from build123d import *

# Parameters (mm, degrees)
SKETCH_1_R          = 2.5
EXTRUDE_1_DEPTH     = 16
SKETCH_2_R          = 4.25
EXTRUDE_2_DEPTH     = 5
SKETCH_3_R          = 2
CUT_EXTRUDE_1_DEPTH = 3.4
CHAMFER_1_SIZE      = 0.8
FILLET_1_R          = 0.4
FILLET_2_R          = 0.2
CHAMFER_2_SIZE      = 0.4
CHAMFER_2_SIZE2     = 0.230940108
CUT_EXTRUDE_2_DEPTH = 2.8


with BuildPart() as part:
    # Эскиз1 → Вытянуть1 (new body)
    with BuildSketch(Plane(origin=(0, 0, 0), x_dir=(0, 0, -1), z_dir=(1, 0, 0))):
        Circle(SKETCH_1_R)
    extrude(amount=EXTRUDE_1_DEPTH)

    # Эскиз2 → Вытянуть2 (add)
    with BuildSketch(Plane.ZY):
        Circle(SKETCH_2_R)
    extrude(amount=EXTRUDE_2_DEPTH)

    # Эскиз3 → Вырез-Вытянуть1 (cut)
    with BuildSketch(Plane.ZY.offset(5)):
        Circle(SKETCH_3_R)
    extrude(amount=-CUT_EXTRUDE_1_DEPTH, mode=Mode.SUBTRACT)

    # Фаска1
    chamfer_1_edges = [part.edges().sort_by_distance(p)[0] for p in [
        (16, 0, 2.5),
    ]]
    chamfer(chamfer_1_edges, length=CHAMFER_1_SIZE)

    # Скругление1
    fillet_1_edges = [part.edges().sort_by_distance(p)[0] for p in [
        (-5, 0, -4.25),
    ]]
    fillet(fillet_1_edges, radius=FILLET_1_R)

    # Скругление2
    fillet_2_edges = [part.edges().sort_by_distance(p)[0] for p in [
        (0, 0, 2.5),
    ]]
    fillet(fillet_2_edges, radius=FILLET_2_R)

    # Фаска2
    chamfer_2_edges = [part.edges().sort_by_distance(p)[0] for p in [
        (-5, 0, -2),
    ]]
    chamfer_2_side = [part.faces().sort_by_distance(p)[0] for p in [
        (-5, 0, -3.741105556),
    ]]
    chamfer(chamfer_2_edges, length=CHAMFER_2_SIZE, length2=CHAMFER_2_SIZE2, reference=chamfer_2_side[0])

    # Эскиз4 → Вырез-Вытянуть2 (cut)
    with BuildSketch(Plane.ZY.offset(5)):
        Polygon((2.309401077, 0), (1.154700538, 2), (-1.154700538, 2), (-2.309401077, 0), (-1.154700538, -2), (1.154700538, -2), align=None)
    extrude(amount=-CUT_EXTRUDE_2_DEPTH, mode=Mode.SUBTRACT)


solid = part.part
Work out the finished part from the listing and answer in its coordinate system (mm). A direction names the side the tool comes from. Round coordinates to 2 decimals unless told otherwise and drop trailing zeros. Loops run counter-clockwise (first coordinate to the right, second up) from the corner with the lowest first, then second, coordinate; pieces in that order, holes last. Notation, with made-up numbers: (-2.5, -40) - (41.5, -40) arc R35 ccw to (41.5, -8) - close; hole circle Ø8 at (-37, -5). An arc over 180 degrees is marked (long way). Use one line per item in the form item = value. Start each with the question number.
(1) Which of the six approach directions +Z, -Z, +X, -X, +Y, -Y give full straight-line access (tool end or side, diameter ignored) to faces 1 (the face through (7.59, -2.44, 0.54)), 2 (the face through (16, 0, 0)), 3 (the face through (-4, -2, 0))?
(2) Find section A-A on x = -2.5. Determine the outline of the cut face in (y, z), and give its area (3 significant figures).
(3) Determine the mould class of faces 4 (the face through (0, -3, 0)), 5 (the face through (-2.268, 3.584, 2.285)), 6 (the face through (-3.593, 1.014, -1.724)) for opening direction Z: +Z half, -Z half, draft (parallel to the pull), parting line (faces both ways), or undercut.
(4) Flat-ended cylindrical pins translate along their axes: P1, Ø3, axis at x = 10, z = -2, coming from the +Y side; P2, Ø4, axis at x = 7, z = 0.5, coming from the +Y side; P3, Ø1.2, axis at x = -4, z = 0.5, coming from the -Y side; P4, Ø3, axis at x = 0.5, y = 2, coming from the +Z side. Find the tip coordinate at first contact, or state that the pin passes through.
(5) Consider line 1 (Y direction, x = -1.85, z = 0); line 2 (Y direction, x = 12.25, z = -1.5); line 3 (X direction, y = -3, z = 2). Determine where each line is inside the solid, lowest interval first.
(6) Find section B-B on x = 8.75. Determine the outline of the cut face in (y, z).
Answer list:
q1.face_1 = +X
q1.face_2 = +Z, -Z, +X, +Y, -Y
q1.face_3 = -X
q2.outline = circle Ø8.5 at (0, 0); hole (-2, -1.15) - (0, -2.31) - (2, -1.15) - (2, 1.15) - (0, 2.31) - (-2, 1.15) - close
q2.area = 42.9 mm^2
q3.face_4 = draft
q3.face_5 = parting line
q3.face_6 = undercut
q4.P1 = 2.45
q4.P2 = 2.5
q4.P3 = -4.25
q4.P4 = 4.21
q5.line_1 = -4.25 to -2, 2 to 4.25
q5.line_2 = -2 to 2
q5.line_3 = -5 to 0
q6.outline = circle Ø5 at (0, 0)
